Read the model definition and answer for the solid it produces. Units are mm, in the model's axes. Face numbers are marked on the shaded views. Round coordinates to 2 decimals unless told otherwise and drop trailing zeros. Order: outer loops, then holes, each group sorted by start corner. A loop starts at its lowest first (then second) coordinate and runs counter-clockwise, first axis right, second up. Notation, with made-up numbers: (50, 56.5) -> (107, 56.5) arc R17 ccw to (107, 73.5) -> close; hole circle Ø5 at (-24, 21). An arc over 180 degrees is marked (long way). Answer as a JSON object with one key per item and string values. Group by question number.
Item 1: The mould has two halves that part along X. Classify the marked faces 1, 2, 3 and 4: pulls with the +X half, pulls with the -X half, needs draft (parallel to the pull), parting line crosses it, or undercut.
Item 2: Section A-A, the plane z = 6.5 is taken. Write down the section's boundary in (x, y).
Item 3: Consider probe 1 along X at (y, z) = (2.4, 6); probe 2 along X at (y, z) = (0.95, 7.5); probe 3 along Z at (x, y) = (0, 0.75). Determine where each line is inside the solid, lowest interval first. Write a range as from..to.
Item 4: Section B-B, the plane y = 1.25 is taken. Write down the section's boundary in (x, z).
Item 5: Section C-C, the plane z = -3.75 is taken. Write down the section's boundary in (x, y), plus the area to 3 significant figures.
Item 6: Section D-D, the plane x = 0 is taken. Write down the section's boundary in (y, z).
Item 7: Given P1, Ø4, axis at x = -11, z = -12, coming from the -Y side; P2, Ø0.9, axis at x = 16.5, y = 2, coming from the -Z side, each flat-ended and moving along its own axis, determine where each tip first touches the part or whether it passes through.
from build123d import *

# Parameters (mm, degrees)
BOSS_EXTRUDE1_DEPTH = 3
SKETCH2_W           = 3
SKETCH2_H           = 3
CUT_EXTRUDE1_DEPTH  = 70.726054689


with BuildPart() as part:
    # Sketch1 → Boss-Extrude1 (new body)
    with BuildSketch(Plane(origin=(0, 0, 0), x_dir=(1, 0, 0), z_dir=(0, 1, 0))):
        with BuildLine():
            Line((-20, 0), (-20, -10))
            Line((-20, -10), (-14, -10))
            Line((-14, -10), (-14, 0))
            ThreePointArc((-14, 0), (0, 14), (14, 0))
            Line((14, 0), (14, -10))
            Line((14, -10), (20, -10))
            Line((20, -10), (20, 0))
            ThreePointArc((20, 0), (0, 20), (-20, 0))
        make_face()
    extrude(amount=BOSS_EXTRUDE1_DEPTH)

    # Sketch2 → Cut-Extrude1 (cut, through all)
    with BuildSketch(Plane(origin=(-39.0910666, 6, -26.523534202), x_dir=(1, 0, 0), z_dir=(0, 1, 0))):
        with Locations((22.0910666, -32.023534202)):
            Rectangle(SKETCH2_W, SKETCH2_H)
        with Locations((56.0910666, -32.023534202)):
            Rectangle(SKETCH2_W, SKETCH2_H)
    extrude(amount=-CUT_EXTRUDE1_DEPTH, mode=Mode.SUBTRACT)


solid = part.part
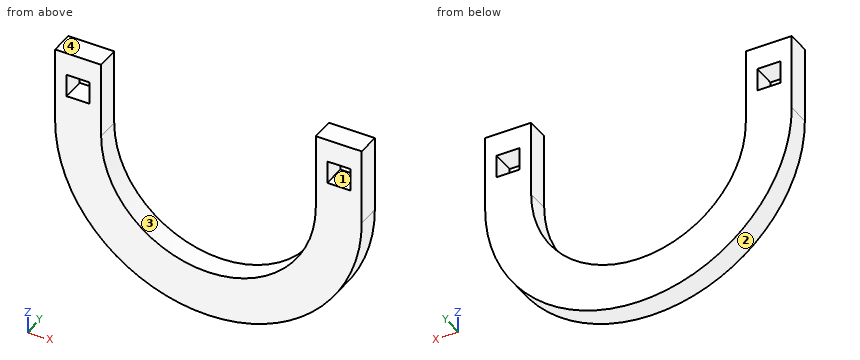
Values found:
{
 "1": {"face 1": "undercut", "face 2": "parting line crosses it", "face 3": "undercut", "face 4": "needs draft"},
 "2": {"outline": "(-20, 0) -> (-18.5, 0) -> (-18.5, 3) -> (-20, 3) -> close; (-15.5, 0) -> (-14, 0) -> (-14, 3) -> (-15.5, 3) -> close; (14, 0) -> (15.5, 0) -> (15.5, 3) -> (14, 3) -> close; (18.5, 0) -> (20, 0) -> (20, 3) -> (18.5, 3) -> close"},
 "3": {"probe 1": "-20..-18.5, -15.5..-14, 14..15.5, 18.5..20", "probe 2": "-20..-14, 14..20", "probe 3": "-20..-14"},
 "4": {"outline": "(-20, 0) arc R20 ccw to (20, 0) -> (20, 10) -> (14, 10) -> (14, 0) arc R14 cw to (-14, 0) -> (-14, 10) -> (-20, 10) -> close; hole (-18.5, 4) -> (-15.5, 4) -> (-15.5, 7) -> (-18.5, 7) -> close; hole (15.5, 4) -> (18.5, 4) -> (18.5, 7) -> (15.5, 7) -> close"},
 "5": {"outline": "(-19.65, 0) -> (-13.49, 0) -> (-13.49, 3) -> (-19.65, 3) -> close; (13.49, 0) -> (19.65, 0) -> (19.65, 3) -> (13.49, 3) -> close", "area": "36.9 mm2"},
 "6": {"outline": "(0, -20) -> (3, -20) -> (3, -14) -> (0, -14) -> close"},
 "7": {"P1": "y = 0", "P2": "z = -11.93"}
}
